Part print with two shaded views. Sizes in mm from the minimum x, y, z corner. A direction names the side the tool comes from. Round coordinates to 2 decimals unless told otherwise and drop trailing zeros. Loops run counter-clockwise (first coordinate to the right, second up) from the corner with the lowest first, then second, coordinate; pieces in that order, holes last. Notation, with made-up numbers: (-11.5, 18) -> (-6.5, 18) arc R32 cw to (-6.5, 57) -> close; hole circle Ø4 at (-32.5, -21.5). An arc over 180 degrees is marked (long way). Answer as a JSON object with one key per item and string values. Group by question number.
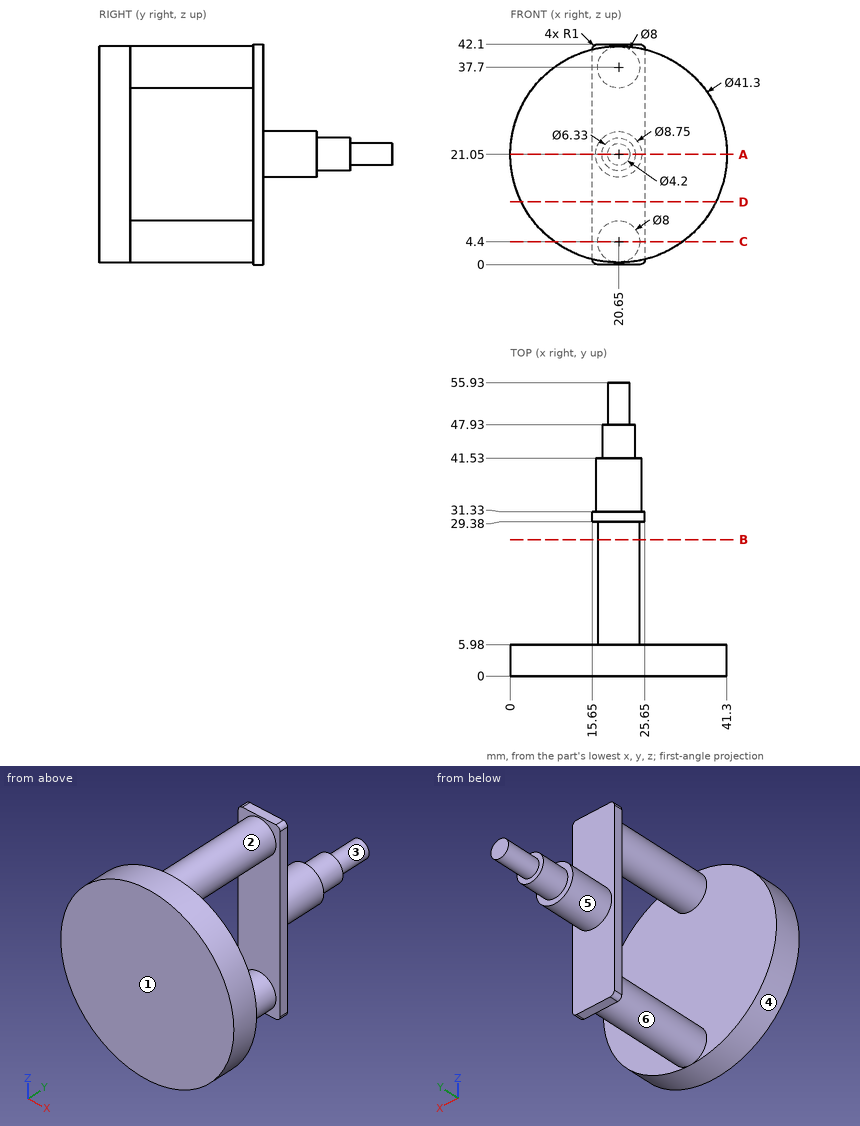
Item 1: Band-saw the part on B-B, the plane y = 26. List the corners of the cut face in (x, z).
Item 2: Band-saw the part on D-D, the plane z = 12. List the corners of the cut face in (x, y), plus the area to 3 significant figures.
Item 3: Drop flat-ended pins along their axis: pin 1 Ø0.6 at (y, z) = (30.5, 25) entering from +X; pin 2 Ø1 at (x, z) = (33, 18) entering from -Y; pin 3 Ø0.6 at (y, z) = (30.5, 28.5) entering from -X; pin 4 Ø3 at (y, z) = (47, 14.5) entering from -X. Give the stop position or say it passes through.
Item 4: Band-saw the part on A-A, the plane z = 21.05. List the corners of the cut face in (x, y) (3 decimals).
Item 5: Drill centre lines: line 1 (Y direction, x = 16, z = 9.5); line 2 (Y direction, x = 26.5, z = 21.5); line 3 (Y direction, x = 21, z = 36). Where is each one in solid material? Low to high.
Item 6: Which spindle directions (+Z, -Z, +X, -X, +Y, -Y) get a long thin tool onto all of the face, cutting with end or side? Do the marked faces 4, 5 and 6. Say none if no direction does.
Item 7: Two-plate mould, pull along Y, no slides. Class the marked faces 1, 2 and 3: pulls with the +Y half, pulls with the -Y half, needs draft (parallel to the pull), parting line crosses it, or undercut.
Item 8: Band-saw the part on C-C, the plane z = 4.4. List the corners of the cut face in (x, y).
Entries:
{
 "1": {"outline": "circle Ø8 at (20.65, 4.4); circle Ø8 at (20.65, 37.7)"},
 "2": {"outline": "(2.09, 0) -> (39.21, 0) -> (39.21, 5.98) -> (2.09, 5.98) -> close; (15.65, 29.38) -> (25.65, 29.38) -> (25.65, 31.33) -> (15.65, 31.33) -> close", "area": "241 mm²"},
 "3": {"pin 1": "x = 25.65", "pin 2": "y = 0", "pin 3": "x = 15.65", "pin 4": "through"},
 "4": {"outline": "(0, 0) -> (41.3, 0) -> (41.3, 5.98) -> (0, 5.98) -> close; (15.65, 29.38) -> (25.65, 29.38) -> (25.65, 31.33) -> (25.025, 31.33) -> (25.025, 41.53) -> (23.815, 41.53) -> (23.815, 47.93) -> (22.75, 47.93) -> (22.75, 55.93) -> (18.55, 55.93) -> (18.55, 47.93) -> (17.485, 47.93) -> (17.485, 41.53) -> (16.275, 41.53) -> (16.275, 31.33) -> (15.65, 31.33) -> close"},
 "5": {"line 1": "0 to 5.98, 29.38 to 31.33", "line 2": "0 to 5.98", "line 3": "0 to 31.33"},
 "6": {"face 4": "-Y", "face 5": "+Y", "face 6": "none"},
 "7": {"face 1": "pulls with the -Y half", "face 2": "undercut", "face 3": "needs draft"},
 "8": {"outline": "(8.44, 0) -> (32.86, 0) -> (32.86, 5.98) -> (24.65, 5.98) -> (24.65, 29.38) -> (25.65, 29.38) -> (25.65, 31.33) -> (15.65, 31.33) -> (15.65, 29.38) -> (16.65, 29.38) -> (16.65, 5.98) -> (8.44, 5.98) -> close"}
}
